Geometry check sheet. Reference: drawing and pictorial views, mm from the part's lowest x, y, z. A direction names the side the tool comes from. Give positions to 0.01 mm unless a question says otherwise; leave off trailing zeros. Write each loop counter-clockwise with the first axis right and the second up, starting at its lowest first coordinate (ties: lowest second). Pieces come first, ordered by that corner, then holes. Notation, with made-up numbers: (21.5, 83.25) -> (26.5, 83.25) arc R17 cw to (26.5, 92.25) -> close; hole circle Ø2 at (46.25, 71.5). An arc over 180 degrees is marked (long way). Return JSON: item names as keys, results as strings.
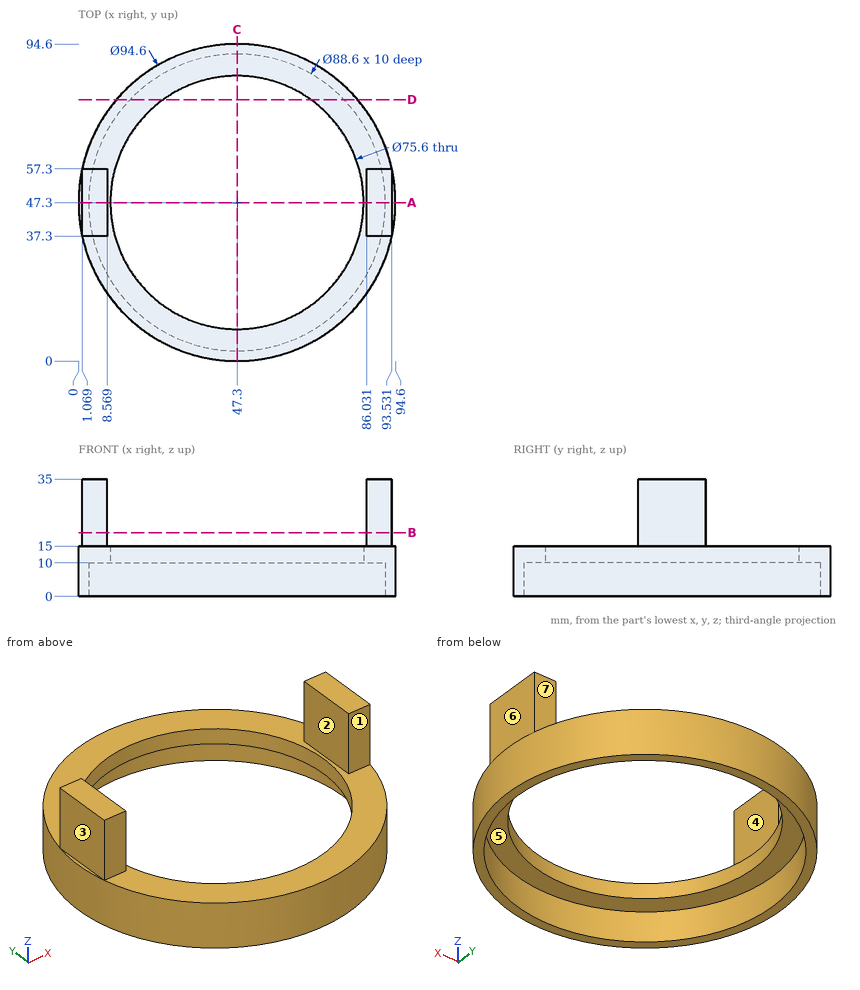
(1) Cross-section at A-A on y = 47.3. Enter the section's corners in (x, z), then the cut area to 3 significant figures.
Reply:
{"outline": "(0, 0) -> (3, 0) -> (3, 10) -> (9.5, 10) -> (9.5, 15) -> (8.57, 15) -> (8.57, 35) -> (1.07, 35) -> (1.07, 15) -> (0, 15) -> close; (85.1, 10) -> (91.6, 10) -> (91.6, 0) -> (94.6, 0) -> (94.6, 15) -> (93.53, 15) -> (93.53, 35) -> (86.03, 35) -> (86.03, 15) -> (85.1, 15) -> close", "area": "455 mm^2"}
(2) Release check for a two-part mould opening along X. For the marked faces 1, 2 and 3 record: pulls with the +X half, pulls with the -X half, needs draft (parallel to the pull), parting line crosses it, or undercut.
Reply:
{"face 1": "needs draft", "face 2": "undercut", "face 3": "pulls with the -X half"}
(3) Set-up check for the marked faces 4, 5, 6 and 7: record each of +Z, -Z, +X, -X, +Y, -Y from which the full face is reachable in a straight line by a thin tool's end or side.
Reply:
{"face 4": "+Z, +Y, -Y", "face 5": "-Z", "face 6": "+Z, +X, +Y, -Y", "face 7": "+Z, +X, -X, +Y"}
(4) Cross-section at C-C on x = 47.3. Enter the section's corners in (y, z).
Reply:
{"outline": "(0, 0) -> (3, 0) -> (3, 10) -> (9.5, 10) -> (9.5, 15) -> (0, 15) -> close; (85.1, 10) -> (91.6, 10) -> (91.6, 0) -> (94.6, 0) -> (94.6, 15) -> (85.1, 15) -> close"}
(5) Thickness scan on L1, parallel to X at y = 47.3, z = 2.75; L2, parallel to Y at x = 47.3, z = 12.7. Record the ranges inside material, lowest first.
Reply:
{"L1": "0 to 3, 91.6 to 94.6", "L2": "0 to 9.5, 85.1 to 94.6"}
(6) Cross-section at B-B on z = 19. Enter the section's corners in (x, y).
Reply:
{"outline": "(1.07, 37.3) -> (8.57, 37.3) -> (8.57, 57.3) -> (1.07, 57.3) -> close; (86.03, 37.3) -> (93.53, 37.3) -> (93.53, 57.3) -> (86.03, 57.3) -> close"}
(7) Cross-section at D-D on y = 78. Enter the section's corners in (x, z).
Reply:
{"outline": "(11.32, 0) -> (15.36, 0) -> (15.36, 10) -> (25.25, 10) -> (25.25, 15) -> (11.32, 15) -> close; (69.35, 10) -> (79.24, 10) -> (79.24, 0) -> (83.28, 0) -> (83.28, 15) -> (69.35, 15) -> close"}
(8) Depth check by flat-ended pin: pin 1 Ø16 at (y, z) = (51.5, 30) entering from -X; pin 2 Ø8 at (x, z) = (6, 22.5) entering from -Y; pin 3 Ø1.5 at (x, z) = (46.5, 17.5) entering from +Y; pin 4 Ø12 at (x, z) = (52, 7) entering from -Y. Enter the tip coordinate at first touch or a pass-through.
Reply:
{"pin 1": "x = 1.07", "pin 2": "y = 37.3", "pin 3": "through", "pin 4": "y = 0"}
